```python
from build123d import *

# Parameters (mm, degrees)
SKETCH1_W           = 100
SKETCH1_H           = 100
BOSS_EXTRUDE1_DEPTH = 35
SKETCH2_W           = 50
SKETCH2_H           = 17.5
CUT_EXTRUDE1_DEPTH  = 30
SKETCH3_R           = 2.5
CUT_EXTRUDE2_DEPTH  = 10
SKETCH4_R           = 3.75
CUT_EXTRUDE3_DEPTH  = 4
SKETCH5_R           = 2.5
CUT_EXTRUDE4_DEPTH  = 30
SKETCH6_R           = 3.75
CUT_EXTRUDE5_DEPTH  = 4
SKETCH7_R           = 2.5
CUT_EXTRUDE10_DEPTH = 79.89866919
SKETCH8_R           = 3.75
CUT_EXTRUDE11_DEPTH = 4
FILLET1_R           = 3


with BuildPart() as part:
    # Sketch1 → Boss-Extrude1 (new body)
    with BuildSketch(Plane(origin=(0, 0, 0), x_dir=(1, 0, 0), z_dir=(0, 1, 0))):
        Rectangle(SKETCH1_W, SKETCH1_H)
    extrude(amount=BOSS_EXTRUDE1_DEPTH)

    # Sketch2 → Cut-Extrude1 (cut)
    with BuildSketch(Plane(origin=(50, 0, 0), x_dir=(0, 0, -1), z_dir=(1, 0, 0))):
        with Locations((0, 17.5)):
            Rectangle(SKETCH2_W, SKETCH2_H)
    cut_extrude1 = extrude(amount=-CUT_EXTRUDE1_DEPTH, mode=Mode.SUBTRACT)

    # Mirror1: Cut-Extrude1 across plane
    add(cut_extrude1.mirror(Plane(origin=(0, 0, 0), x_dir=(0, 0, 1), z_dir=(1, 0, 0))), mode=Mode.SUBTRACT)

    # Sketch3 → Cut-Extrude2 (cut)
    with BuildSketch(Plane(origin=(0, 35, 0), x_dir=(1, 0, 0), z_dir=(0, 1, 0))):
        with Locations(Location((35, 12.5, 0), (0, 0, 270))):
            Circle(SKETCH3_R)
        with Locations(Location((35, -12.5, 0), (0, 0, 270))):
            Circle(SKETCH3_R)
        with Locations(Location((-35, -12.5, 0), (0, 0, 270))):
            Circle(SKETCH3_R)
        with Locations(Location((-35, 12.5, 0), (0, 0, 90))):
            Circle(SKETCH3_R)
    extrude(amount=-CUT_EXTRUDE2_DEPTH, mode=Mode.SUBTRACT)

    # Sketch4 → Cut-Extrude3 (cut)
    with BuildSketch(Plane(origin=(0, 35, 0), x_dir=(1, 0, 0), z_dir=(0, 1, 0))):
        with Locations(Location((35, 12.5, 0), (0, 0, 270))):
            Circle(SKETCH4_R)
        with Locations(Location((35, -12.5, 0), (0, 0, 90))):
            Circle(SKETCH4_R)
        with Locations(Location((-35, -12.5, 0), (0, 0, 270))):
            Circle(SKETCH4_R)
        with Locations(Location((-35, 12.5, 0), (0, 0, 90))):
            Circle(SKETCH4_R)
    extrude(amount=-CUT_EXTRUDE3_DEPTH, mode=Mode.SUBTRACT)

    # Sketch5 → Cut-Extrude4 (cut)
    with BuildSketch(Plane(origin=(0, 0, -50), x_dir=(-1, 0, 0), z_dir=(0, 0, -1))):
        with Locations((-35, 17.5)):
            Circle(SKETCH5_R)
        with Locations(Location((35, 17.5, 0), (0, 0, 270))):
            Circle(SKETCH5_R)
    cut_extrude4 = extrude(amount=-CUT_EXTRUDE4_DEPTH, mode=Mode.SUBTRACT)

    # Sketch6 → Cut-Extrude5 (cut)
    with BuildSketch(Plane(origin=(0, 0, -50), x_dir=(-1, 0, 0), z_dir=(0, 0, -1))):
        with Locations((-35, 17.5)):
            Circle(SKETCH6_R)
        with Locations(Location((35, 17.5, 0), (0, 0, 180))):
            Circle(SKETCH6_R)
    cut_extrude5 = extrude(amount=-CUT_EXTRUDE5_DEPTH, mode=Mode.SUBTRACT)

    # Mirror2: Cut-Extrude4, Cut-Extrude5 across plane
    add(cut_extrude4.mirror(Plane.XY), mode=Mode.SUBTRACT)
    add(cut_extrude5.mirror(Plane.XY), mode=Mode.SUBTRACT)

    # Sketch7 → Cut-Extrude10 (cut, through all)
    with BuildSketch(Plane(origin=(0, 35, 0), x_dir=(1, 0, 0), z_dir=(0, 1, 0))):
        with Locations(Location((5, 30, 0), (0, 0, 270))):
            Circle(SKETCH7_R)
        with Locations(Location((5, -30, 0), (0, 0, 90))):
            Circle(SKETCH7_R)
        with Locations(Location((-5, -30, 0), (0, 0, 270))):
            Circle(SKETCH7_R)
        with Locations(Location((-5, 30, 0), (0, 0, 90))):
            Circle(SKETCH7_R)
    extrude(amount=-CUT_EXTRUDE10_DEPTH, mode=Mode.SUBTRACT)

    # Sketch8 → Cut-Extrude11 (cut)
    with BuildSketch(Plane(origin=(0, 35, 0), x_dir=(1, 0, 0), z_dir=(0, 1, 0))):
        with Locations(Location((-5, 30, 0), (0, 0, 270))):
            Circle(SKETCH8_R)
        with Locations(Location((5, 30, 0), (0, 0, 90))):
            Circle(SKETCH8_R)
        with Locations(Location((5, -30, 0), (0, 0, 270))):
            Circle(SKETCH8_R)
        with Locations(Location((-5, -30, 0), (0, 0, 90))):
            Circle(SKETCH8_R)
    extrude(amount=-CUT_EXTRUDE11_DEPTH, mode=Mode.SUBTRACT)

    # Fillet1
    fillet1_edges = [part.edges().sort_by_distance(p)[0] for p in [
        (0, 35, 50),
        (0, 35, -50),
    ]]
    fillet(fillet1_edges, radius=FILLET1_R)


solid = part.part
```
Source: CAD feature listing. Evaluate the final solid. Frame: model axes, mm. A direction names the side the tool comes from. Coordinates: 2 decimals unless noted, no trailing zeros. Loops run counter-clockwise (first coordinate to the right, second up) from the corner with the lowest first, then second, coordinate; pieces in that order, holes last. Notation, with made-up numbers: M 40,-33 L 96,-33 A22 cw 96,-25 Z; hole C 68.5,57 d9. An arc over 180 degrees is marked long. Put each result on its own line as item: value. Start each with the question number.
1) Contact query for flat-ended pins moving along their axis: pin 1 Ø6 at (x, z) = (-35, -12.5) entering from +Y; pin 2 Ø4 at (x, y) = (36.5, 18) entering from -Z; pin 3 Ø1.5 at (y, z) = (23, -18) entering from +X. Output: stop coordinate, or through.
2) Cut plane B-B on x = -5. Return the cut outline in (y, z).
3) Pull-direction query (Z, two-part tool) for faces 1 (the face through (32.615, 18.251, 35.647)), 2 (the face through (34, 15, -46)), 3 (the face through (-35, 8.75, 0)); classes: pulls with the +Z half, pulls with the -Z half, needs draft (parallel to the pull), parting line crosses it, or undercut.
4) Cut plane C-C on z = -12.5. Return the cut outline in (x, y), then the cut area to 3 significant figures.
5) Cut plane A-A on z = -30. Return the cut outline in (x, y), then the cut area to 3 significant figures.
6) Ray query, L1, parallel to Z at x = 45, y = 18; L2, parallel to Y at x = -34.5, z = -19; L3, parallel to X at y = 26, z = -29. Return the intervals inside material, ascending. Write a range as from..to.
7) Reachability of faces 4 (the face through (35.81, 13.84, 48.03)), 5 (the face through (-20, 18, 0)), 6 (the face through (39, 17, 25)), 7 (the face through (-33.27, 20.827, -48.028)), 8 (the face through (-33, 29, 11)) from +Z, -Z, +X, -X, +Y, -Y: full face, straight path, thin tool, end or side. Return the list, or none.
8) Cut plane D-D on y = 17.5. Give the number of separate pieces and of enclosed holes in the cut face, then the cut area to 3 significant figures.
The answers:
1. pin 1: stops at y = 31
1. pin 2: stops at z = -46
1. pin 3: stops at x = 20
2. outline: M 0,-50 L 32,-50 A3 ccw 35,-47 L 35,-33.75 L 31,-33.75 L 31,-32.5 L 0,-32.5 Z; M 0,-27.5 L 31,-27.5 L 31,-26.25 L 35,-26.25 L 35,26.25 L 31,26.25 L 31,27.5 L 0,27.5 Z; M 0,32.5 L 31,32.5 L 31,33.75 L 35,33.75 L 35,47 A3 ccw 32,50 L 0,50 Z
3. face 1: needs draft
3. face 2: pulls with the -Z half
3. face 3: undercut
4. outline: M -50,0 L 50,0 L 50,8.75 L 20,8.75 L 20,26.25 L 32.5,26.25 L 32.5,31 L 31.25,31 L 31.25,35 L -31.25,35 L -31.25,31 L -32.5,31 L -32.5,26.25 L -20,26.25 L -20,8.75 L -50,8.75 Z; M -50,26.25 L -37.5,26.25 L -37.5,31 L -38.75,31 L -38.75,35 L -50,35 Z; M 37.5,26.25 L 50,26.25 L 50,35 L 38.75,35 L 38.75,31 L 37.5,31 Z
4. area: 2,340 mm²
5. outline: M -50,0 L -7.5,0 L -7.5,31 L -8.75,31 L -8.75,35 L -50,35 Z; M -2.5,0 L 2.5,0 L 2.5,31 L 1.25,31 L 1.25,35 L -1.25,35 L -1.25,31 L -2.5,31 Z; M 7.5,0 L 50,0 L 50,35 L 8.75,35 L 8.75,31 L 7.5,31 Z; hole C -35,17.5 d5; hole C 35,17.5 d5
5. area: 3,090 mm²
6. L1: z = -50..-25, 25..50
6. L2: y = 0..8.75, 26.25..35
6. L3: x = -50..-7.29, -2.71..2.71, 7.29..50
7. face 4: +Z
7. face 5: -X
7. face 6: +X
7. face 7: -Z
7. face 8: +Y
8. separate pieces: 5
8. enclosed holes: 4
8. area: 6,380 mm²
